Can you work these out from the model? Positions are in its coordinate system, mm. Face numbers are marked on the shaded views. A direction names the side the tool comes from. Coordinates: 2 decimals unless noted, no trailing zeros. Order: outer loops, then holes, each group sorted by start corner. A loop starts at its lowest first (then second) coordinate and runs counter-clockwise, first axis right, second up. Notation, with made-up numbers: (-11, 86) -> (12, 86) arc R12 cw to (12, 95) -> close; hole circle Ø1 at (-18, 60). An arc over 180 degrees is marked (long way). Answer in a Markdown table with one row per item. Add a question column.
1. We'd pull the mould along X, two halves only. Please class the marked faces 5, 6 and 7: pulls with the +X half, pulls with the -X half, needs draft (parallel to the pull), parting line crosses it, or undercut.
2. Imagine slicing it at D-D on x = -26. Write out the boundary of the cut face in (y, z) (3 decimals), plus the area to 3 significant figures.
3. Imagine slicing it at A-A on y = 14.5. Write out the boundary of the cut face in (x, z).
4. Imagine slicing it at B-B on x = 0. Write out the boundary of the cut face in (y, z) (3 decimals), plus the area to 3 significant figures.
5. Imagine slicing it at C-C on z = -11. Write out the boundary of the cut face in (x, y).
6. Will these pins go through, and if not, where does the flat tip stop? pin 1 (3 mm diameter, centred on x = 9, y = 4.5, fed in from +Z); pin 2 (1.5 mm diameter, centred on y = 2, z = -11.5, fed in from -X); pin 3 (7.5 mm diameter, centred on x = 40.5, y = 17, fed in from +Z); pin 4 (23.5 mm diameter, centred on x = 38, z = 5.5, fed in from +Y).
7. On a 3-axis mill with a long thin cutter (end or side, diameter ignored), from which of +Z, -Z, +X, -X, +Y, -Y can I reach the whole of each face in a straight line? I mean the marked faces 1, 2, 3 and 4. Say none if no direction works.
8. If I drill on line 1 along X through (y, z) = (19.5, -17); line 2 along X through (y, z) = (10.5, -13); line 3 along Z through (x, y) = (-20.5, 4), over which ranges is the centre line in solid material (lowest first)? Write a range as [from, to].
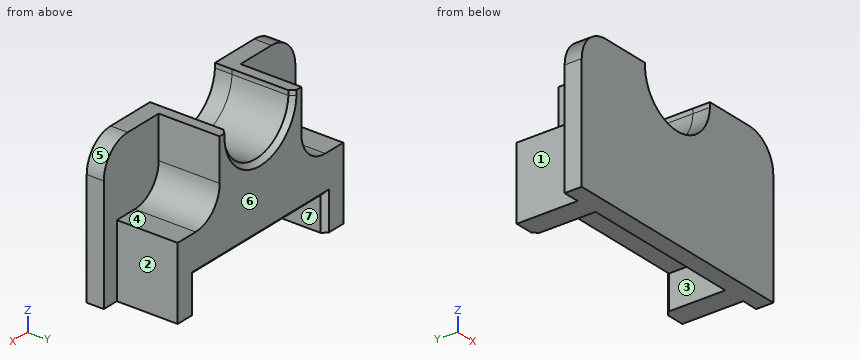
from build123d import *

# Parameters (mm, degrees)
F1_DEPTH = 7.112
F3_DEPTH = 25.4
F4_SIZE  = 1.905
F5_DEPTH = 25.4
F6_SIZE  = 1.905


with BuildPart() as f1:
    # F0 (on Front) → F1 (new body)
    with BuildSketch(Plane.XZ):
        with BuildLine():
            Line((-50.8, -30.2332285792), (50.8, -30.2332285792))
            Line((50.8, -30.2332285792), (50.8, 17.5332285792))
            ThreePointArc((50.8, 17.5332285792), (47.0802561211, 26.5134847002), (38.1, 30.2332285792))
            Line((38.1, 30.2332285792), (-38.1, 30.2332285792))
            ThreePointArc((-38.1, 30.2332285792), (-47.0802561211, 26.5134847002), (-50.8, 17.5332285792))
            Line((-50.8, 17.5332285792), (-50.8, -30.2332285792))
        make_face()
    extrude(amount=F1_DEPTH)

    # F2 (on Front) → F3 (join)
    with BuildSketch(Plane.XZ):
        with BuildLine():
            Line((-43.9048968256, 0), (-43.9048968256, -30.2332285792))
            Line((-43.9048968256, -30.2332285792), (-34.3798968256, -30.2332285792))
            Line((-34.3798968256, -30.2332285792), (-34.3798968256, -16.0933099687))
            Line((-34.3798968256, -16.0933099687), (0, -16.0933099687))
            Line((0, -16.0933099687), (34.3798968256, -16.0933099687))
            Line((34.3798968256, -16.0933099687), (34.3798968256, -30.2332285792))
            Line((34.3798968256, -30.2332285792), (43.9048968256, -30.2332285792))
            Line((43.9048968256, -30.2332285792), (43.9048968256, 0))
            Line((43.9048968256, 0), (34.3798968256, 0))
            ThreePointArc((34.3798968256, 0), (25.3996407045, 3.7197438789), (21.6798968256, 12.7))
            Line((21.6798968256, 12.7), (21.6798968256, 30.2332285792))
            Line((21.6798968256, 30.2332285792), (17.2348968256, 30.2332285792))
            ThreePointArc((17.2348968256, 30.2332285792), (17.2625602078, 29.2563374186), (17.2348968256, 28.2794462581))
            ThreePointArc((17.2348968256, 28.2794462581), (0, 11.9937772108), (-17.2348968256, 28.2794462581))
            ThreePointArc((-17.2348968256, 28.2794462581), (-17.2625602078, 29.2563374186), (-17.2348968256, 30.2332285792))
            Line((-17.2348968256, 30.2332285792), (-21.6798968256, 30.2332285792))
            Line((-21.6798968256, 30.2332285792), (-21.6798968256, 12.7))
            ThreePointArc((-21.6798968256, 12.7), (-25.3996407045, 3.7197438789), (-34.3798968256, 0))
            Line((-34.3798968256, 0), (-43.9048968256, 0))
        make_face()
    extrude(amount=-F3_DEPTH)

    # F4
    f4_edges = [f1.edges().sort_by_distance(p)[0] for p in [
        (34.379897, 25.4, -23.163269),
        (0, 25.4, -16.09331),
        (-34.379897, 25.4, -23.163269),
    ]]
    chamfer(f4_edges, length=F4_SIZE)

    # F5 (cut): a face of the model
    f5_faces = [f1.faces().sort_by_distance(p)[0] for p in [
        (0, 0, 22.4548498087),
    ]]
    extrude(f5_faces, amount=-F5_DEPTH, mode=Mode.SUBTRACT)

    # F6
    f6_edges = [f1.edges().sort_by_distance(p)[0] for p in [
        (0.976891, 25.4, 12.021441),
    ]]
    chamfer(f6_edges, length=F6_SIZE)


solid = f1.part
Answers follow:
| question | item | result |
|---|---|---|
| 1 | face 5 | pulls with the +X half |
| 1 | face 6 | needs draft |
| 1 | face 7 | undercut |
| 2 | outline | (-7.112, -30.233) -> (0, -30.233) -> (0, -16.093) -> (23.495, -16.093) -> (25.4, -14.188) -> (25.4, 3.157) -> (0, 3.157) -> (0, 30.233) -> (-7.112, 30.233) -> close |
| 2 | area | 917 mm² |
| 3 | outline | (-43.9, -30.23) -> (-34.38, -30.23) -> (-34.38, -16.09) -> (34.38, -16.09) -> (34.38, -30.23) -> (43.9, -30.23) -> (43.9, 0) -> (34.38, 0) arc R12.7 cw to (21.68, 12.7) -> (21.68, 30.23) -> (17.23, 30.23) arc R17.26 cw (long way) to (-17.23, 30.23) -> (-21.68, 30.23) -> (-21.68, 12.7) arc R12.7 cw to (-34.38, 0) -> (-43.9, 0) -> close |
| 4 | outline | (-7.112, -30.233) -> (0, -30.233) -> (0, -16.093) -> (23.495, -16.093) -> (25.4, -14.188) -> (25.4, 10.089) -> (23.495, 11.994) -> (-7.112, 11.994) -> close |
| 4 | area | 1,010 mm² |
| 5 | outline | (-50.8, -7.11) -> (50.8, -7.11) -> (50.8, 0) -> (43.9, 0) -> (43.9, 25.4) -> (-43.9, 25.4) -> (-43.9, 0) -> (-50.8, 0) -> close |
| 6 | pin 1 | stops at z = 15.55 |
| 6 | pin 2 | stops at x = -43.9 |
| 6 | pin 3 | stops at z = 0 |
| 6 | pin 4 | stops at y = 25.4 |
| 7 | face 1 | +Z, -Z, -X, +Y |
| 7 | face 2 | +Z, -Z, +X, +Y |
| 7 | face 3 | -Z, +Y |
| 7 | face 4 | +Z, +X, +Y |
| 8 | line 1 | x = [-43.9, -34.38], [34.38, 43.9] |
| 8 | line 2 | x = [-43.9, 43.9] |
| 8 | line 3 | z = [-16.09, 30.23] |
